Design review of the part built by this model. Coordinates are the model's own, in mm. A direction names the side the tool comes from. Round coordinates to 2 decimals unless told otherwise and drop trailing zeros. Order: outer loops, then holes, each group sorted by start corner. A loop starts at its lowest first (then second) coordinate and runs counter-clockwise, first axis right, second up. Notation, with made-up numbers: M 66,-11 L 96,-11 A37 ccw 96,25 Z; hole C -18,-28.75 d5. An arc over 180 degrees is marked long. Write each question's results on one line, items separated by ' | '. Start each with the question number.
Item 1: Take a section at D-D, the plane z = 7.5. Write out the cut boundary in (x, y).
Item 2: Machinability: for faces 1 (the flat face through (19, -1, 0)), 2 (the flat face through (-28, -1, 0)), 3 (the flat face through (-10, -1, 8)), 4 (the flat face through (-13, -20, 12)), which of the approach directions +Z, -Z, +X, -X, +Y, -Y give a long, thin tool a straight path to every point of the face, cutting with its end or side? Answer none if there is none.
Item 3: Clearance check with flat-ended pins moving along their axes: pin 1 (11.5 mm diameter, centred on x = 16.5, y = -4, fed in from +Z); pin 2 (6 mm diameter, centred on y = -13.5, z = 17, fed in from -X); pin 3 (3 mm diameter, centred on y = -25, z = 12, fed in from +X). State where each tip first meets the part, or that it passes through.
Item 4: Wall thickness on line 1 (X direction, y = -12.5, z = 18.25); line 2 (Z direction, x = -0.5, y = -7); line 3 (Z direction, x = -13, y = -8): over which ranges is each line inside the solid? List them lowest first. Write a range as [from, to].
Item 5: The part is to be moulded in two halves that separate along Y. For faces 5 (the flat face through (-13, 0, 10)), 6 (the flat face through (-5, -40, -1)), 7 (the cylindrical face through (-12, 0, 18)), 8 (the flat face through (-5, -1, 0)), say which applies: +Y half, -Y half, draft (parallel to the pull), parting line (faces both ways), or undercut.
Item 6: Take a section at C-C, the plane y = -13.5. Write out the cut boundary in (x, z).
Item 7: Take a section at A-A, the plane z = 14. Write out the cut boundary in (x, y).
Item 8: Take a section at B-B, the plane x = 2. Write out the cut boundary in (y, z), plus the area to 3 significant figures.
```python
from build123d import *

# Parameters (mm, degrees)
F0_W     = 5
F0_H     = 20
F1_DEPTH = 40
F2_R     = 2
F3_R     = 2
F4_W     = 40
F4_H     = 5
F5_DEPTH = 25
F6_R     = 10
F7_DEPTH = 25


with BuildPart() as f1:
    # F0 (on Front) → F1 (new body, symmetric)
    with BuildSketch(Plane.XZ):
        with Locations((-12.5, 10)):
            Rectangle(F0_W, F0_H)
        Polygon((0, 0), (-10, 0), (-15, 0), (-40, 0), (-40, -5), (0, -5), align=None)
        with Locations((2.5, 10)):
            Rectangle(F0_W, F0_H)
        Polygon((5, 0), (0, 0), (0, -5), (30, -5), (30, 0), align=None)
    extrude(amount=F1_DEPTH, both=True)

    # F2
    f2_edges = [f1.edges().sort_by_distance(p)[0] for p in [
        (5, 0, 0),
        (-15, 0, 0),
    ]]
    fillet(f2_edges, radius=F2_R)

    # F3
    f3_edges = [f1.edges().sort_by_distance(p)[0] for p in [
        (-15, 0, 20),
        (5, 0, 20),
    ]]
    fillet(f3_edges, radius=F3_R)

    # F4 (on face) → F5 (cut)
    with BuildSketch(Plane(origin=(-15, 0, 0), x_dir=(0, -1, 0), z_dir=(-1, 0, 0))):
        with Locations((0, 12.5)):
            Rectangle(F4_W, F4_H)
    extrude(amount=-F5_DEPTH, mode=Mode.SUBTRACT)

    # F6 (on face) → F7 (cut)
    with BuildSketch(Plane.YZ.offset(5)):
        with Locations((0, 28)):
            Circle(F6_R)
    extrude(amount=-F7_DEPTH, mode=Mode.SUBTRACT)


solid = f1.part
```
Results list:
1) outline: M -15,-40 L -10,-40 L -10,40 L -15,40 Z; M 0,-40 L 5,-40 L 5,40 L 0,40 Z
2) face 1: +Z, +X, +Y, -Y | face 2: +Z, -X, +Y, -Y | face 3: +Z, +Y, -Y | face 4: +X, -X
3) pin 1: z = 0 | pin 2: x = -15 | pin 3: x = 5
4) line 1: [-14.98, -10], [0, 4.98] | line 2: [-5, 0] | line 3: [-5, 10], [15, 20]
5) face 5: undercut | face 6: -Y half | face 7: undercut | face 8: draft
6) outline: M -40,-5 L 30,-5 L 30,0 L 7,0 A2 cw 5,2 L 5,10 L 0,10 L 0,0 L -10,0 L -10,10 L -15,10 L -15,2 A2 cw -17,0 L -40,0 Z; M -15,15 L -10,15 L -10,20 L -13,20 A2 ccw -15,18 Z; M 0,15 L 5,15 L 5,18 A2 ccw 3,20 L 0,20 Z
7) outline: M -15,-40 L -10,-40 L -10,-20 L -15,-20 Z; M -15,20 L -10,20 L -10,40 L -15,40 Z; M 0,-40 L 5,-40 L 5,-20 L 0,-20 Z; M 0,20 L 5,20 L 5,40 L 0,40 Z
8) outline: M -40,-5 L 40,-5 L 40,20 L 6,20 A10 cw -6,20 L -40,20 Z; hole M -20,10 L 20,10 L 20,15 L -20,15 Z | area: 1,780 mm²
